Can you work these out from the model? Positions are in its coordinate system, mm. A direction names the side the tool comes from. Give positions to 0.01 mm unless a question says otherwise; leave off trailing zeros. Loops run counter-clockwise (first coordinate to the right, second up) from the corner with the lowest first, then second, coordinate; pieces in that order, holes last. Notation, with made-up numbers: (41.25, 13.25) - (56.25, 13.25) arc R21 cw to (56.25, 31.25) - close; hole circle Ø6 at (-23.75, 5.5). An arc over 180 degrees is marked (long way). Answer as a JSON object with one key per item and string values. Group by question number.
Item 1: Suppose I cut it at C-C on y = 41.5. Write out the boundary of the cut face in (x, z), and give its area (3 significant figures).
Item 2: Suppose I cut it at A-A on y = 13. Write out the boundary of the cut face in (x, z), and give its area (3 significant figures).
Item 3: Will these pins go through, and if not, where does the flat tip stop? pin 1 (1 mm diameter, centred on x = -171, z = -85.5, fed in from +Y); pin 2 (4.5 mm diameter, centred on x = -132.5, z = 15, fed in from +Y); pin 3 (0.7 mm diameter, centred on x = -131, y = 15.5, fed in from +Z).
Item 4: Which directions (+Z, -Z, +X, -X, +Y, -Y) give clear straight access to the entire face, cutting with the end or side of a thin tool? Please do faces 4 (the cylindrical face through (-121.904, 32.65, -129.93)), 5 (the flat face through (-134, 11, -60)), 6 (the flat face through (-159, 33, -125)).
Item 5: Suppose I cut it at D-D on x = -146. Write out the boundary of the cut face in (y, z).
Item 6: Please list where these lines run through material, in increasing order: L1, parallel to Z at x = -104, y = 34; L2, parallel to X at y = 43.5, z = -125.5; L3, parallel to Z at x = -175, y = 17.5.
Item 7: Thinking about a two-plate mould opening in X: for faces 1 (the flat face through (-91, 45.046, -106)), 2 (the flat face through (-159, 33, 35)), 3 (the flat face through (-85, 2, -44)), which applies, pulls with the +X half, pulls with the -X half, needs draft (parallel to the pull), parting line crosses it, or undercut?
Item 8: Suppose I cut it at B-B on z = -100.5. Write out the boundary of the cut face in (x, y).
from build123d import *

# Parameters (mm, degrees)
BOSS_EXTRUDE1_DEPTH     = 15.045877519
BOSS_EXTRUDE2_DEPTH     = 30
BOSS_EXTRUDE3_DEPTH     = 160
CUT_EXTRUDE1_DEPTH      = 397.42670329
CUT_EXTRUDE1_DEPTH_BACK = 397.42670329
SKETCH5_W               = 30
SKETCH5_H               = 30
CUT_EXTRUDE2_START      = -30
CUT_EXTRUDE2_DEPTH      = 30
CUT_EXTRUDE3_DEPTH      = 10
CUT_EXTRUDE4_DEPTH      = 263.019333412


# Read off the part's stored shape, not the designer's step: Boss-Extrude3
with BuildPart() as part:
    # Sketch1 → Boss-Extrude1 (new body)
    with BuildSketch(Plane(origin=(0, 0, 0), x_dir=(1, 0, 0), z_dir=(0, 1, 0))):
        with BuildLine():
            Line((-185, -65), (5, -65))
            ThreePointArc((5, -65), (60.514401442, -84.704810384), (91.182336182, -135))
            Line((91.182336182, -135), (185, -135))
            Line((185, -135), (185, 135))
            Line((185, 135), (-185, 135))
            Line((-185, 135), (-185, -65))
        make_face()
    extrude(amount=BOSS_EXTRUDE1_DEPTH)

    # Sketch2 → Boss-Extrude2 (add)
    with BuildSketch(Plane(origin=(0, 15.045877519, 0), x_dir=(1, 0, 0), z_dir=(0, 1, 0))):
        Polygon((-175, -35), (-175, 30), (-185, 30), (-185, -45), (-142.5, -45), (-142.5, -35), align=None)
        Polygon((-175, 125), (-142.5, 125), (-142.5, 135), (-185, 135), (-185, 60), (-175, 60), align=None)
        Polygon((-95, -35), (-95, 30), (-85, 30), (-85, -45), (-127.5, -45), (-127.5, -35), align=None)
        Polygon((-127.5, 135), (-127.5, 125), (-95, 125), (-95, 60), (-85, 60), (-85, 135), align=None)
    extrude(amount=BOSS_EXTRUDE2_DEPTH)

    # Boss-Extrude3 outline → Boss-Extrude3 (add)
    with BuildSketch(Plane.XY.offset(-125)):
        with BuildLine():
            ThreePointArc((-95, 45.045877519), (-110, 23.379210852), (-135, 15.045877519))
            Line((-135, 15.045877519), (-95, 15.045877519))
            Line((-95, 15.045877519), (-95, 45.045877519))
        make_face()
        with BuildLine():
            Line((-175, 45.045877519), (-175, 15.045877519))
            Line((-175, 15.045877519), (-135, 15.045877519))
            ThreePointArc((-135, 15.045877519), (-160, 23.379210852), (-175, 45.045877519))
        make_face()
    extrude(amount=BOSS_EXTRUDE3_DEPTH)

    # Sketch5 → Cut-Extrude1 (cut, two sides: drawn at the far end of the back side and taken through both)
    with BuildSketch(Plane.ZY.offset(185).offset(-CUT_EXTRUDE1_DEPTH_BACK)):
        with Locations((-45, 30.045877519)):
            Rectangle(SKETCH5_W, SKETCH5_H)
    extrude(amount=CUT_EXTRUDE1_DEPTH + CUT_EXTRUDE1_DEPTH_BACK, mode=Mode.SUBTRACT)

    # Sketch6 → Cut-Extrude2 (cut)
    with BuildSketch(Plane(origin=(0, 15.045877519, 0), x_dir=(1, 0, 0), z_dir=(0, 1, 0)).offset(CUT_EXTRUDE2_START)):
        with BuildLine():
            Line((-142.5, -45), (-127.5, -45))
            Line((-127.5, -45), (-85, -45))
            Line((-85, -45), (-85, 30))
            Line((-85, 30), (-85, 60))
            Line((-85, 60), (-85, 135))
            Line((-85, 135), (185, 135))
            Line((185, 135), (185, -135))
            Line((185, -135), (91.182336182, -135))
            ThreePointArc((91.182336182, -135), (60.514401442, -84.704810384), (5, -65))
            Line((5, -65), (-185, -65))
            Line((-185, -65), (-185, -45))
            Line((-185, -45), (-142.5, -45))
        make_face()
    extrude(amount=CUT_EXTRUDE2_DEPTH, mode=Mode.SUBTRACT)

    # Sketch8 → Cut-Extrude3 (cut)
    with BuildSketch(Plane(origin=(0, 15.045877519, 0), x_dir=(1, 0, 0), z_dir=(0, 1, 0))):
        Polygon((-135, 30), (-85, 30), (-85, 60), (-135, 60), (-185, 60), (-185, 30), align=None)
    extrude(amount=-CUT_EXTRUDE3_DEPTH, mode=Mode.SUBTRACT)

    # Sketch9 → Cut-Extrude4 (cut, through all)
    with BuildSketch(Plane.XY.offset(45)):
        with BuildLine():
            Line((-150, 45.045877519), (-120, 45.045877519))
            ThreePointArc((-120, 45.045877519), (-123.28072965, 28.827812568), (-132.437534993, 15.045877519))
            Line((-132.437534993, 15.045877519), (-137.562465007, 15.045877519))
            ThreePointArc((-137.562465007, 15.045877519), (-146.71927035, 28.827812568), (-150, 45.045877519))
        make_face()
    extrude(amount=-CUT_EXTRUDE4_DEPTH, mode=Mode.SUBTRACT)


solid = part.part
Worked out:
{
 "1": {"outline": "(-185, -135) - (-149.83, -135) - (-149.83, -125) - (-173.79, -125) - (-173.79, -60) - (-185, -60) - close; (-185, -30) - (-173.79, -30) - (-173.79, 35) - (-149.83, 35) - (-149.83, 45) - (-185, 45) - close; (-120.17, -135) - (-85, -135) - (-85, -60) - (-96.21, -60) - (-96.21, -125) - (-120.17, -125) - close; (-120.17, 35) - (-96.21, 35) - (-96.21, -30) - (-85, -30) - (-85, 45) - (-120.17, 45) - close", "area": "4,320 mm2"},
 "2": {"outline": "(-185, -135) - (-85, -135) - (-85, -60) - (-185, -60) - close; (-185, -30) - (-85, -30) - (-85, 45) - (-185, 45) - close", "area": "15,000 mm2"},
 "3": {"pin 1": "stops at y = 36.62", "pin 2": "stops at y = 15.32", "pin 3": "stops at z = 35"},
 "4": {"face 4": "+Z, -Z, +Y", "face 5": "+X, -X, +Y", "face 6": "+Y"},
 "5": {"outline": "(0, -135) - (27.19, -135) - (27.19, -125) - (16.52, -125) - (16.52, -60) - (5.05, -60) - (5.05, -30) - (16.52, -30) - (16.52, 35) - (27.19, 35) - (27.19, 45) - (0, 45) - close"},
 "6": {"L1": "z = -135 to -125, 35 to 45", "L2": "x = -185 to -149.96, -120.04 to -85", "L3": "z = -135 to -60, -30 to 45"},
 "7": {"face 1": "needs draft", "face 2": "undercut", "face 3": "pulls with the +X half"},
 "8": {"outline": "(-185, 0) - (-85, 0) - (-85, 45.05) - (-95, 45.05) arc R41.67 cw to (-132.35, 15.13) arc R43.04 cw to (-132.44, 15.05) - (-137.56, 15.05) arc R43.04 cw to (-137.65, 15.13) arc R41.67 cw to (-175, 45.05) - (-185, 45.05) - close"}
}
